```python
from build123d import *

# Parameters (mm, degrees)
SKETCH1_R           = 14.2875
BOSS_EXTRUDE1_DEPTH = 3.175
FILLET1_R           = 2.54


with BuildPart() as part:
    # Sketch1 → Boss-Extrude1 (new body)
    with BuildSketch(Plane.XY):
        with BuildLine():
            Line((25.4, -19.05), (19.05, -19.05))
            Line((19.05, -19.05), (19.05, -57.15))
            Line((19.05, -57.15), (-19.05, -57.15))
            Line((-19.05, -57.15), (-19.05, -19.05))
            Line((-19.05, -19.05), (-19.05, -12.7))
            ThreePointArc((-19.05, -12.7), (-9.750640303, 9.750640303), (12.7, 19.05))
            Line((12.7, 19.05), (25.4, 19.05))
            ThreePointArc((25.4, 19.05), (44.45, 0), (25.4, -19.05))
        make_face()
        with Locations((25.4, 0)):
            Circle(SKETCH1_R, mode=Mode.SUBTRACT)
        with Locations((0, -38.1)):
            Circle(SKETCH1_R, mode=Mode.SUBTRACT)
    extrude(amount=BOSS_EXTRUDE1_DEPTH)

    # Fillet1
    fillet1_edges = [part.edges().sort_by_distance(p)[0] for p in [
        (19.05, -19.05, 1.5875),
        (19.05, -57.15, 1.5875),
        (-19.05, -57.15, 1.5875),
    ]]
    fillet(fillet1_edges, radius=FILLET1_R)


solid = part.part
```
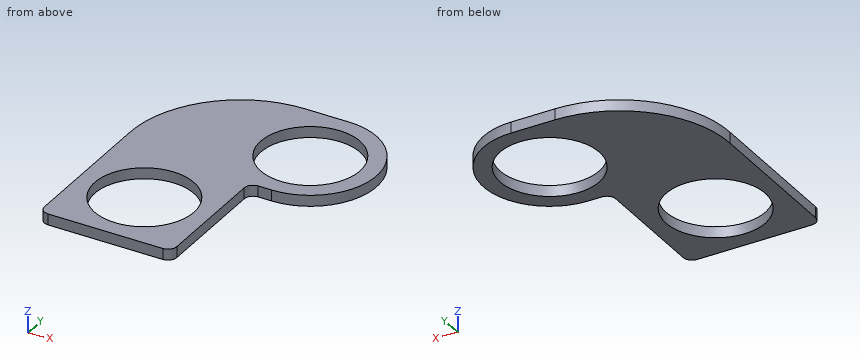
Could you check a few things on this model? Use its own coordinates, in mm. Coordinates: 2 decimals unless noted, no trailing zeros. Write each loop counter-clockwise with the first axis right and the second up, starting at its lowest first coordinate (ties: lowest second). Pieces come first, ordered by that corner, then holes. Notation, with made-up numbers: (25.5, 9.25) -> (78.5, 9.25) arc R16 ccw to (78.5, 14.25) -> close; hole circle Ø11 at (89, -29.5). An arc over 180 degrees is marked (long way). Write item = value, one per line. Start each with the question number.
(1) Will these pins go through, and if not, where does the flat tip stop? pin 1 (1 mm diameter, centred on y = -45, z = 2, fed in from +X); pin 2 (2 mm diameter, centred on x = 0.5, y = -10.5, fed in from -Z); pin 3 (10 mm diameter, centred on x = 4.5, y = -40.5, fed in from -Z).
(2) I want a section at B-B (x = -3). Please give me the cut outline in (y, z) (3 decimals), plus the area to 3 significant figures.
(3) I want a section at A-A (z = 2). Give the number of separate pieces and of enclosed holes in the cut face, plus the area to 3 significant figures.
(4) I need wall thicknesses on line 1 (X direction, y = -46.5, z = 3); line 2 (X direction, y = -41, z = 1.95); line 3 (Y direction, x = 26, z = 0.1). Which ranges of each line are inside material? Lowest first, please. Write a range as [from, to].
Result set:
q1.pin_1 = 19.05
q1.pin_2 = 0
q1.pin_3 = through
q2.outline = (-57.15, 0) -> (-52.069, 0) -> (-52.069, 3.175) -> (-57.15, 3.175) -> close; (-24.131, 0) -> (14.897, 0) -> (14.897, 3.175) -> (-24.131, 3.175) -> close
q2.area = 140 mm2
q3.separate_pieces = 1
q3.enclosed_holes = 2
q3.area = 2,210 mm2
q4.line_1 = [-19.05, -11.56], [11.56, 19.05]
q4.line_2 = [-19.05, -13.99], [13.99, 19.05]
q4.line_3 = [-19.04, -14.27], [14.27, 19.04]
